Check sheet for the drawn part. Datum: minimum x, y, z corner. Units: mm. A direction names the side the tool comes from. Give positions to 0.01 mm unless a question says otherwise; leave off trailing zeros. Order: outer loops, then holes, each group sorted by start corner. A loop starts at its lowest first (then second) coordinate and runs counter-clockwise, first axis right, second up. Notation, with made-up numbers: M 40.5,-3 L 83.5,-3 A30 ccw 83.5,32 Z; hole C 55,82.25 d9. An arc over 180 degrees is marked long. Put each result on its own line as item: value. Start each with the question number.
Q1. Section check A-A on y = 71.5. Record the cut outline in (x, z).
Q2. Material ranges on L1, parallel to X at y = 63.5, z = 0.45; L2, parallel to Y at x = 7.5, z = 1.3; L3, parallel to Y at x = 4.25, z = 2.7, recorded low to high.
Q3. Go/stop test with flat-tipped pins: pin 1 (1.2 mm diameter, centred on x = 22, z = 3.5, fed in from -Y); pin 2 (2.5 mm diameter, centred on x = 17, z = 3.5, fed in from +Y). Record where each tip stops, or that it passes through.
Q4. Section check B-B on x = 19.25. Record the cut outline in (y, z), then the cut area to 3 significant figures.
Q5. Access from +Z, -Z, +X, -X, +Y, -Y to the whole of each face (thin tool, end or side, straight path). Record for the marked faces 1, 2 and 3.
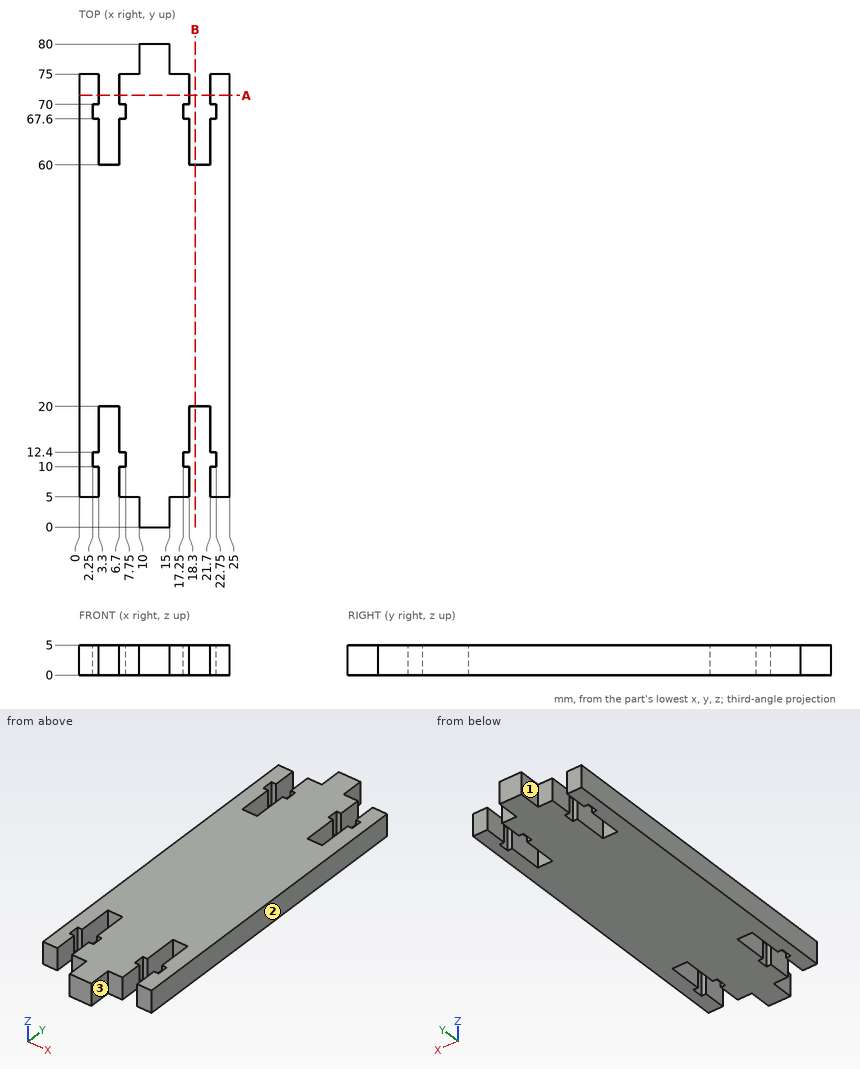
Results found:
1. outline: M 0,0 L 3.3,0 L 3.3,5 L 0,5 Z; M 6.7,0 L 18.3,0 L 18.3,5 L 6.7,5 Z; M 21.7,0 L 25,0 L 25,5 L 21.7,5 Z
2. L1: x = 0 to 3.3, 6.7 to 18.3, 21.7 to 25
2. L2: y = 5 to 10, 12.4 to 67.6, 70 to 75
2. L3: y = 20 to 60
3. pin 1: stops at y = 5
3. pin 2: stops at y = 75
4. outline: M 20,0 L 60,0 L 60,5 L 20,5 Z
4. area: 200 mm^2
5. face 1: +Z, -Z, -X, +Y
5. face 2: +Z, -Z, +X, +Y, -Y
5. face 3: +Z, -Z, +X, -Y
